The drawing under review shows one solid part. Ordinate dimensions are in mm from its lowest x, y, z. A direction names the side the tool comes from. Coordinates: 2 decimals unless noted, no trailing zeros. Write each loop counter-clockwise with the first axis right and the second up, starting at its lowest first coordinate (ties: lowest second). Pieces come first, ordered by that corner, then holes.
Q1. Add section A-A, the plane x = 5. Give the boundary of the cut face in (y, z), plus the area to 3 significant figures.
Q2. Add section B-B, the plane y = 8.75. Give the boundary of the cut face in (x, z), plus the area to 3 significant figures.
Q3. To check wall thickness, follow probe 1 along X at (y, z) = (0.8, 17); probe 2 along Y at (x, z) = (20.5, 23.5); probe 3 along Y at (x, z) = (12, 21). State the ranges of each line that lie inside material, in increasing order.
Q4. Add section D-D, the plane x = 2.25. Give the boundary of the cut face in (y, z).
Q5. Machinability: for the marked faces 1, 2, 3 and 4, which of the approach directions +Z, -Z, +X, -X, +Y, -Y give a long, thin tool a straight path to every point of the face, cutting with its end or side? Answer none if there is none.
Q6. Clearance check with flat-ended pins moving along their axes: pin 1 Ø12 at (x, z) = (8.5, 21.5) entering from +Y; pin 2 Ø8 at (y, z) = (13.5, 9.5) entering from -X; pin 3 Ø0.9 at (x, y) = (20, 8) entering from +Z. State where each tip first meets the part, or that it passes through.
Q7. Add section C-C, the plane y = 12. Give the boundary of the cut face in (x, z), plus the area to 3 significant figures.
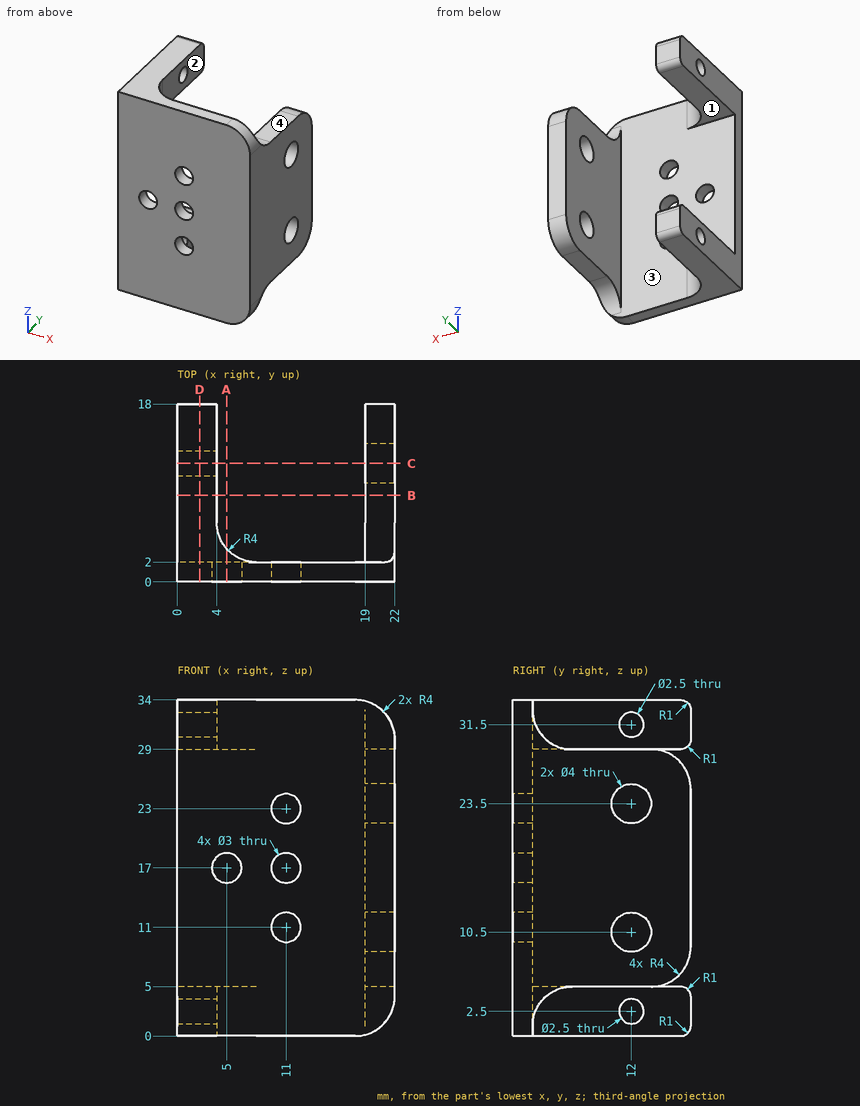
Here are the results:
1. outline: (0, 0) - (3.35, 0) - (3.35, 5) - (2, 5) - (2, 15.5) - (0, 15.5) - close; (0, 18.5) - (2, 18.5) - (2, 29) - (3.35, 29) - (3.35, 34) - (0, 34) - close
1. area: 75.5 mm2
2. outline: (0, 0) - (4, 0) - (4, 5) - (0, 5) - close; (0, 29) - (4, 29) - (4, 34) - (0, 34) - close; (19, 5) - (22, 5) - (22, 29) - (19, 29) - close
2. area: 112 mm2
3. probe 1: x = 0 to 3.5, 6.5 to 9.5, 12.5 to 22
3. probe 2: y = 0 to 10, 14 to 18
3. probe 3: y = 0 to 2
4. outline: (0, 0) - (17, 0) arc R1 ccw to (18, 1) - (18, 4) arc R1 ccw to (17, 5) - (2, 5) - (2, 29) - (17, 29) arc R1 ccw to (18, 30) - (18, 33) arc R1 ccw to (17, 34) - (0, 34) - close; hole circle Ø2.5 at (12, 2.5); hole circle Ø2.5 at (12, 31.5)
5. face 1: -X, +Y
5. face 2: +Z, -Z, +X, +Y
5. face 3: +Y
5. face 4: +Z, +X, +Y
6. pin 1: stops at y = 2
6. pin 2: stops at x = 19
6. pin 3: stops at z = 29
7. outline: (0, 0) - (4, 0) - (4, 1.25) - (0, 1.25) - close; (0, 3.75) - (4, 3.75) - (4, 5) - (0, 5) - close; (0, 29) - (4, 29) - (4, 30.25) - (0, 30.25) - close; (0, 32.75) - (4, 32.75) - (4, 34) - (0, 34) - close; (19, 5) - (22, 5) - (22, 8.5) - (19, 8.5) - close; (19, 12.5) - (22, 12.5) - (22, 21.5) - (19, 21.5) - close; (19, 25.5) - (22, 25.5) - (22, 29) - (19, 29) - close
7. area: 68.0 mm2
